Job drawing, mm, ordinate dimensions from the low corner. One solid piece. Give positions to 0.01 mm unless a question says otherwise; leave off trailing zeros. Order: outer loops, then holes, each group sorted by start corner. A loop starts at its lowest first (then second) coordinate and runs counter-clockwise, first axis right, second up. Notation, with made-up numbers: (-13, 15) - (6, 15) arc R12 cw to (6, 25) - close; hole circle Ø6 at (-10.75, -11.75). An arc over 180 degrees is marked (long way). Write each question's results on one line, items separated by ' | '. Start each with the question number.
1) Cut at C-C on x = 16. List the corners of the cut face in (y, z).
2) Cut at A-A on z = 31.75. List the corners of the cut face in (x, y), plus the area to 3 significant figures.
3) Cut at B-B on y = 4.25. List the corners of the cut face in (x, z) (3 decimals), plus the area to 3 significant figures.
4) Drill centre lines: line 1 along Z through (x, y) = (13, 2.5); line 2 along X through (y, z) = (4.25, 31.75); line 3 along X through (y, z) = (4, 41) (3 decimals). Where is each one in solid material? Low to high. Write a range as from..to.
5) Drop flat-ended pins along their axis: pin 1 Ø3 at (x, y) = (55, 3) entering from +Z; pin 2 Ø1 at (y, z) = (1.5, 6.5) entering from +X. Give the stop position or say it passes through.
6) Cut at D-D on x = 51.5. List the corners of the cut face in (y, z).
7) Two-plate mould, pull along X, no slides. Class the marked faces 1, 2 and 3: +X half, -X half, draft (parallel to the pull), parting line (faces both ways), or undercut.
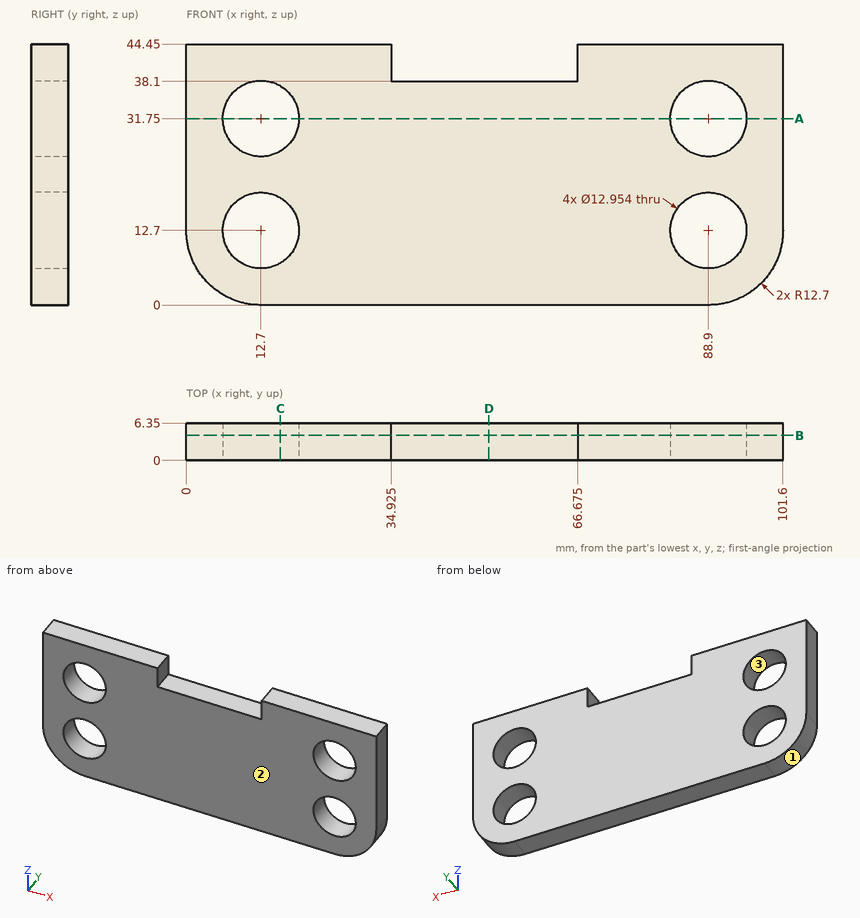
Results:
1) outline: (0, 0) - (6.35, 0) - (6.35, 7.13) - (0, 7.13) - close; (0, 18.27) - (6.35, 18.27) - (6.35, 26.18) - (0, 26.18) - close; (0, 37.32) - (6.35, 37.32) - (6.35, 44.45) - (0, 44.45) - close
2) outline: (0, 0) - (6.22, 0) - (6.22, 6.35) - (0, 6.35) - close; (19.18, 0) - (82.42, 0) - (82.42, 6.35) - (19.18, 6.35) - close; (95.38, 0) - (101.6, 0) - (101.6, 6.35) - (95.38, 6.35) - close | area: 481 mm^2
3) outline: (0, 12.7) arc R12.7 ccw to (12.7, 0) - (88.9, 0) arc R12.7 ccw to (101.6, 12.7) - (101.6, 44.45) - (66.675, 44.45) - (66.675, 38.1) - (34.925, 38.1) - (34.925, 44.45) - (0, 44.45) - close; hole circle Ø12.954 at (12.7, 12.7); hole circle Ø12.954 at (12.7, 31.75); hole circle Ø12.954 at (88.9, 12.7); hole circle Ø12.954 at (88.9, 31.75) | area: 3,720 mm^2
4) line 1: 0..6.23, 19.17..25.28, 38.22..44.45 | line 2: 0..6.22, 19.18..82.42, 95.38..101.6 | line 3: 0..34.925, 66.675..101.6
5) pin 1: z = 38.1 | pin 2: x = 100.25
6) outline: (0, 0) - (6.35, 0) - (6.35, 38.1) - (0, 38.1) - close
7) face 1: -X half | face 2: draft | face 3: undercut
